Build history of the part. All positions in model axes, mm. A direction names the side the tool comes from. Round coordinates to 2 decimals unless told otherwise and drop trailing zeros. Loops run counter-clockwise (first coordinate to the right, second up) from the corner with the lowest first, then second, coordinate; pieces in that order, holes last. Notation, with made-up numbers: M 27.5,14.25 L 84.5,14.25 A23 cw 84.5,28.25 Z; hole C 35,-3 d8. An arc over 180 degrees is marked long. One line per item, written item: value.
```python
from build123d import *

# Parameters (mm, degrees)
BOSS_EXTRUDE1_DEPTH = 10
SKETCH2_W           = 39
SKETCH2_H           = 48.5
BOSS_EXTRUDE2_DEPTH = 10
SKETCH6_R           = 1
BOSS_EXTRUDE3_DEPTH = 4
SKETCH7_W           = 10
SKETCH7_H           = 8.25
CUT_EXTRUDE1_DEPTH  = 10
SKETCH8_R           = 2.25
CUT_EXTRUDE2_DEPTH  = 15
CUT_EXTRUDE3_DEPTH  = 2


with BuildPart() as part:
    # Sketch1 → Boss-Extrude1 (new body)
    with BuildSketch(Plane(origin=(0, 0, 0), x_dir=(1, 0, 0), z_dir=(0, 1, 0))):
        with BuildLine():
            Line((-17.5, 32.5), (17.5, 32.5))
            ThreePointArc((17.5, 32.5), (24.571067812, 29.571067812), (27.5, 22.5))
            Line((27.5, 22.5), (27.5, -22.5))
            ThreePointArc((27.5, -22.5), (24.571067812, -29.571067812), (17.5, -32.5))
            Line((17.5, -32.5), (-17.5, -32.5))
            ThreePointArc((-17.5, -32.5), (-24.571067812, -29.571067812), (-27.5, -22.5))
            Line((-27.5, -22.5), (-27.5, 22.5))
            ThreePointArc((-27.5, 22.5), (-24.571067812, 29.571067812), (-17.5, 32.5))
        make_face()
    extrude(amount=BOSS_EXTRUDE1_DEPTH)

    # Sketch2 → Boss-Extrude2 (add)
    with BuildSketch(Plane(origin=(0, 10, 0), x_dir=(1, 0, 0), z_dir=(0, 1, 0))):
        with BuildLine():
            Line((27.5, 22.5), (27.5, -22.5))
            ThreePointArc((27.5, -22.5), (24.571067812, -29.571067812), (17.5, -32.5))
            Line((17.5, -32.5), (-17.5, -32.5))
            ThreePointArc((-17.5, -32.5), (-24.571067812, -29.571067812), (-27.5, -22.5))
            Line((-27.5, -22.5), (-27.5, 22.5))
            ThreePointArc((-27.5, 22.5), (-24.571067812, 29.571067812), (-17.5, 32.5))
            Line((-17.5, 32.5), (17.5, 32.5))
            ThreePointArc((17.5, 32.5), (24.571067812, 29.571067812), (27.5, 22.5))
        make_face()
        Rectangle(SKETCH2_W, SKETCH2_H, mode=Mode.SUBTRACT)
    extrude(amount=BOSS_EXTRUDE2_DEPTH)

    # Sketch6 → Boss-Extrude3 (add)
    with BuildSketch(Plane(origin=(0, 10, 0), x_dir=(1, 0, 0), z_dir=(0, 1, 0))):
        with Locations(Location((-14, 13.25, 0), (0, 0, 90))):
            Circle(SKETCH6_R)
        with Locations(Location((14, 13.25, 0), (0, 0, 90))):
            Circle(SKETCH6_R)
        with Locations(Location((14, -9.75, 0), (0, 0, 90))):
            Circle(SKETCH6_R)
        with Locations(Location((-14, -9.75, 0), (0, 0, 90))):
            Circle(SKETCH6_R)
    extrude(amount=BOSS_EXTRUDE3_DEPTH)

    # Sketch7 → Cut-Extrude1 (cut)
    with BuildSketch(Plane(origin=(0, 20, 0), x_dir=(1, 0, 0), z_dir=(0, 1, 0))):
        with Locations((0, -28.375)):
            Rectangle(SKETCH7_W, SKETCH7_H)
    extrude(amount=-CUT_EXTRUDE1_DEPTH, mode=Mode.SUBTRACT)

    # Sketch8 → Cut-Extrude2 (cut)
    with BuildSketch(Plane(origin=(0, 20, 0), x_dir=(1, 0, 0), z_dir=(0, 1, 0))):
        with Locations(Location((-21.5, -26, 0), (0, 0, 270))):
            Circle(SKETCH8_R)
        with Locations(Location((21.5, -26, 0), (0, 0, 270))):
            Circle(SKETCH8_R)
        with Locations(Location((21.5, 26, 0), (0, 0, 270))):
            Circle(SKETCH8_R)
        with Locations(Location((-21.5, 26, 0), (0, 0, 270))):
            Circle(SKETCH8_R)
    extrude(amount=-CUT_EXTRUDE2_DEPTH, mode=Mode.SUBTRACT)

    # Sketch9 → Cut-Extrude3 (cut)
    with BuildSketch(Plane(origin=(0, 20, 0), x_dir=(1, 0, 0), z_dir=(0, 1, 0))):
        with BuildLine():
            Line((-14, 28), (14, 28))
            ThreePointArc((14, 28), (16.757724491, 27.612229483), (19.301576132, 26.478991126))
            ThreePointArc((19.301576132, 26.478991126), (19.96113246, 24.358541291), (22.119681664, 23.83701719))
            ThreePointArc((22.119681664, 23.83701719), (23.518319616, 21.066201507), (24, 18))
            Line((24, 18), (24, -18))
            ThreePointArc((24, -18), (23.518319616, -21.066201507), (22.119681664, -23.83701719))
            ThreePointArc((22.119681664, -23.83701719), (19.96113246, -24.358541291), (19.301576132, -26.478991126))
            ThreePointArc((19.301576132, -26.478991126), (16.757724491, -27.612229483), (14, -28))
            Line((14, -28), (-14, -28))
            ThreePointArc((-14, -28), (-16.757724491, -27.612229483), (-19.301576132, -26.478991126))
            ThreePointArc((-19.301576132, -26.478991126), (-19.96113246, -24.358541291), (-22.119681664, -23.83701719))
            ThreePointArc((-22.119681664, -23.83701719), (-23.518319616, -21.066201507), (-24, -18))
            Line((-24, -18), (-24, 18))
            ThreePointArc((-24, 18), (-23.518319616, 21.066201507), (-22.119681664, 23.83701719))
            ThreePointArc((-22.119681664, 23.83701719), (-19.96113246, 24.358541291), (-19.301576132, 26.478991126))
            ThreePointArc((-19.301576132, 26.478991126), (-16.757724491, 27.612229483), (-14, 28))
        make_face()
        with BuildLine():
            Line((-11.5, 26), (11.5, 26))
            ThreePointArc((11.5, 26), (18.571067812, 23.071067812), (21.5, 16))
            Line((21.5, 16), (21.5, -16))
            ThreePointArc((21.5, -16), (18.571067812, -23.071067812), (11.5, -26))
            Line((11.5, -26), (-11.5, -26))
            ThreePointArc((-11.5, -26), (-18.571067812, -23.071067812), (-21.5, -16))
            Line((-21.5, -16), (-21.5, 16))
            ThreePointArc((-21.5, 16), (-18.571067812, 23.071067812), (-11.5, 26))
        make_face(mode=Mode.SUBTRACT)
    extrude(amount=-CUT_EXTRUDE3_DEPTH, mode=Mode.SUBTRACT)


solid = part.part
```
Item 1: Slice it at A-A, the plane y = 9.25. Give the cut face in (x, z), and give its area (3 significant figures).
Check values:
outline: M -27.5,-22.5 A10 ccw -17.5,-32.5 L 17.5,-32.5 A10 ccw 27.5,-22.5 L 27.5,22.5 A10 ccw 17.5,32.5 L -17.5,32.5 A10 ccw -27.5,22.5 Z; hole C -21.5,-26 d4.5; hole C -21.5,26 d4.5; hole C 21.5,-26 d4.5; hole C 21.5,26 d4.5
area: 3,430 mm2
Item 2: Pull direction X, two halves, no side cores. Call faces 3 (the face through (0, 8, 32.5)), 4 (the face through (22, 5, -26)): pulls with the +X half, pulls with the -X half, needs draft (parallel to the pull), parting line crosses it, or undercut.
Check values:
face 3: needs draft
face 4: undercut
Item 3: Slice it at B-B, the plane z = -13.25. Give the cut face in (x, y), and give its area (3 significant figures).
Check values:
outline: M -27.5,0 L 27.5,0 L 27.5,20 L 24,20 L 24,18 L 21.5,18 L 21.5,20 L 19.5,20 L 19.5,10 L 15,10 L 15,14 L 13,14 L 13,10 L -13,10 L -13,14 L -15,14 L -15,10 L -19.5,10 L -19.5,20 L -21.5,20 L -21.5,18 L -24,18 L -24,20 L -27.5,20 Z
area: 716 mm2
Item 4: Slice it at D-D, the plane y = 16.25. Give the cut face in (x, z), and give its area (3 significant figures).
Check values:
outline: M -27.5,-22.5 A10 ccw -17.5,-32.5 L 17.5,-32.5 A10 ccw 27.5,-22.5 L 27.5,22.5 A10 ccw 17.5,32.5 L 5,32.5 L 5,24.25 L 19.5,24.25 L 19.5,-24.25 L -19.5,-24.25 L -19.5,24.25 L -5,24.25 L -5,32.5 L -17.5,32.5 A10 ccw -27.5,22.5 Z; hole C -21.5,-26 d4.5; hole C -21.5,26 d4.5; hole C 21.5,-26 d4.5; hole C 21.5,26 d4.5
area: 1,450 mm2
Item 5: Which spindle directions (+Z, -Z, +X, -X, +Y, -Y) get a long thin tool onto all of the face, cutting with end or side? Do faces 1 (the face through (21.5, 19, 0)), 2 (the face through (-10, 20, 25)). Say none if no direction does.
Check values:
face 1: +Y
face 2: +Z, -Z, +X, -X, +Y
Item 6: Wall check: line 1 along Z through (x, y) = (-21.5, 8.5); line 2 along X through (y, z) = (10.5, 26); line 3 along Z through (x, y) = (15.5, 14.25). Give the ranges that are in metal, low to high.
Check values:
line 1: z = -31.67 to -28.25, -23.75 to 23.75, 28.25 to 31.67
line 2: x = -26.87 to -23.75, -19.25 to -5, 5 to 19.25, 23.75 to 26.87
line 3: z = -32.5 to -24.25, 24.25 to 32.5
Item 7: Slice it at C-C, the plane x = 2.5. Give the cut face in (y, z), and give its area (4 significant figures).
Check values:
outline: M 0,-32.5 L 20,-32.5 L 20,-28 L 18,-28 L 18,-26 L 20,-26 L 20,-24.25 L 10,-24.25 L 10,32.5 L 0,32.5 Z
area: 728.5 mm2
Item 8: Drop flat-ended pins along their axis: P1, Ø2, axis at x = -21.5, y = 9, coming from the +Z side; P2, Ø2, axis at x = 0, y = 13.5, coming from the +Z side; P3, Ø1.6, axis at x = 14.5, z = 9.5, coming from the +Y side. Give the stop position or say it passes through.
Check values:
P1: stops at z = 32.04
P2: stops at z = -24.25
P3: stops at y = 14
